Could you check a few things on this model? Use its own coordinates, in mm. Face numbers are marked on the shaded views. A direction names the side the tool comes from. Coordinates: 2 decimals unless noted, no trailing zeros. Loops run counter-clockwise (first coordinate to the right, second up) from the corner with the lowest first, then second, coordinate; pieces in that order, holes last. Notation, with made-up numbers: M -32.75,7.5 L 2.25,7.5 A11 ccw 2.25,19.5 Z; hole C 10.25,1 d8. An arc over 180 degrees is marked long. Write each question's results on one line, items separated by ' | '.
```python
from build123d import *

# Parameters (mm, degrees)
BOSS_EXTRUDE1_DEPTH      = 54
BOSS_EXTRUDE1_DEPTH_BACK = 46
SKETCH1_R                = 15
BOSS_EXTRUDE3_REACH      = 99.568
SKETCH20_R               = 12.5
SKETCH20_R_2             = 10
SKETCH20_3_R             = 10
CUT_EXTRUDE2_DEPTH       = 20
SKETCH22_R               = 12.5
CUT_EXTRUDE3_DEPTH       = 95
CUT_EXTRUDE6_DEPTH       = 24
CUT_EXTRUDE7_REACH       = 125.735
SKETCH23_R               = 2.435


with BuildPart() as part:
    # Sketch1 → Boss-Extrude1 (new, two sides: drawn at the far end of the back side and taken through both)
    with BuildSketch(Plane.XY.offset(-BOSS_EXTRUDE1_DEPTH_BACK)):
        Circle(SKETCH1_R)
    extrude(amount=BOSS_EXTRUDE1_DEPTH + BOSS_EXTRUDE1_DEPTH_BACK)

    # Loft1: read off the stored shape, not the designer's step
    # Loft1: loft between two sections, ruled curve by curve
    loft1_from = [
        Edge.make_line((-13.008298755, 7.468879668, 18.132780083), (-13.008298755, 7.468879668, -18.132780083)),
        Edge.make_line((-13.008298755, 7.468879668, -18.132780083), (13.008298755, 7.468879668, -18.132780083)),
        Edge.make_line((13.008298755, 7.468879668, 18.132780083), (-13.008298755, 7.468879668, 18.132780083)),
        Edge.make_line((13.008298755, 7.468879668, -18.132780083), (13.008298755, 7.468879668, 18.132780083)),
    ]
    loft1_to = [
        Edge.make_line((-7, 30, 12.5), (-7, 30, -12.5)),
        Edge.make_line((-7, 30, -12.5), (7, 30, -12.5)),
        Edge.make_line((7, 30, 12.5), (-7, 30, 12.5)),
        Edge.make_line((7, 30, -12.5), (7, 30, 12.5)),
    ]
    loft1 = Solid(Shell([*[Face.make_surface_from_curves(loft1_from[k], loft1_to[k]) for k in range(4)], Face(Wire(loft1_from)), Face(Wire(loft1_to))]))
    add(loft1)

    # Boss-Extrude3: up to this plane
    boss_extrude3_end = Plane(origin=(-14.004149378, 3.734439834, 0), z_dir=(0.9662349396012463, -0.25766265056033255, 0))
    # Sketch20 → Boss-Extrude3 (add, up to the surface)
    with BuildSketch(Plane(origin=(32.065513698, 51.244565683, 0), x_dir=(0, 0, -1), z_dir=(0.9063077870366495, 0.4226182617407006, 0)), mode=Mode.PRIVATE) as boss_extrude3_sk1:
        with Locations(Location((0, 0, 0), (0, 0, 90))):
            Circle(SKETCH20_R)
        Circle(SKETCH20_R_2, mode=Mode.SUBTRACT)
    boss_extrude3_tool1 = split(extrude(boss_extrude3_sk1.sketch, amount=-BOSS_EXTRUDE3_REACH, mode=Mode.PRIVATE), bisect_by=boss_extrude3_end, keep=Keep.BOTH, mode=Mode.PRIVATE)
    add(boss_extrude3_tool1.solids().sort_by_distance((37.198824, 40.236147, 0))[0])
    # Sketch20 → Boss-Extrude3 (add, up to the surface)
    with BuildSketch(Plane(origin=(32.065513698, 51.244565683, 0), x_dir=(0, 0, -1), z_dir=(0.9063077870366495, 0.4226182617407006, 0)), mode=Mode.PRIVATE) as boss_extrude3_sk2:
        Circle(SKETCH20_R_2)
    boss_extrude3_tool2 = split(extrude(boss_extrude3_sk2.sketch, amount=-BOSS_EXTRUDE3_REACH, mode=Mode.PRIVATE), bisect_by=boss_extrude3_end, keep=Keep.BOTH, mode=Mode.PRIVATE)
    add(boss_extrude3_tool2.solids().sort_by_distance((32.065514, 51.244566, 0))[0])

    # Sketch20<3> → Cut-Extrude2 (cut)
    with BuildSketch(Plane(origin=(32.065513698, 51.244565683, 0), x_dir=(0, 0, -1), z_dir=(0.9063077870366495, 0.4226182617407006, 0))):
        with Locations(Location((0, 0, 0), (0, 0, 90))):
            Circle(SKETCH20_3_R)
    extrude(amount=-CUT_EXTRUDE2_DEPTH, mode=Mode.SUBTRACT)

    # Sketch22 → Cut-Extrude3 (cut)
    with BuildSketch(Plane(origin=(0, 0, -46), x_dir=(-1, 0, 0), z_dir=(0, 0, -1))):
        Circle(SKETCH22_R)
    extrude(amount=-CUT_EXTRUDE3_DEPTH, mode=Mode.SUBTRACT)

    # Sketch22<3> → Cut-Extrude6 (cut)
    with BuildSketch(Plane(origin=(0, 0, -46), x_dir=(-1, 0, 0), z_dir=(0, 0, -1))):
        with BuildLine():
            ThreePointArc((12.5, 0), (0, -12.5), (-12.5, 0))
            Line((-12.5, 0), (-15, 0))
            ThreePointArc((-15, 0), (0, -15), (15, 0))
            Line((15, 0), (12.5, 0))
        make_face()
    extrude(amount=-CUT_EXTRUDE6_DEPTH, mode=Mode.SUBTRACT)

    # Sketch23 → Cut-Extrude7 (cut, up to next)
    with BuildSketch(Plane.XY.offset(54), mode=Mode.PRIVATE) as cut_extrude7_sk1:
        with Locations((2.172182, -4.201728854)):
            Circle(SKETCH23_R)
    cut_extrude7_tool1 = extrude(cut_extrude7_sk1.sketch, amount=-CUT_EXTRUDE7_REACH, mode=Mode.PRIVATE) & part.part
    add(cut_extrude7_tool1.solids().sort_by_distance((2.172182, -4.201729, 54))[0], mode=Mode.SUBTRACT)


with BuildPart() as body_2:
    # Mirror1: mirrored copy
    add(part.part.mirror(Plane.XY.offset(54)))


solid = body_2.part
```
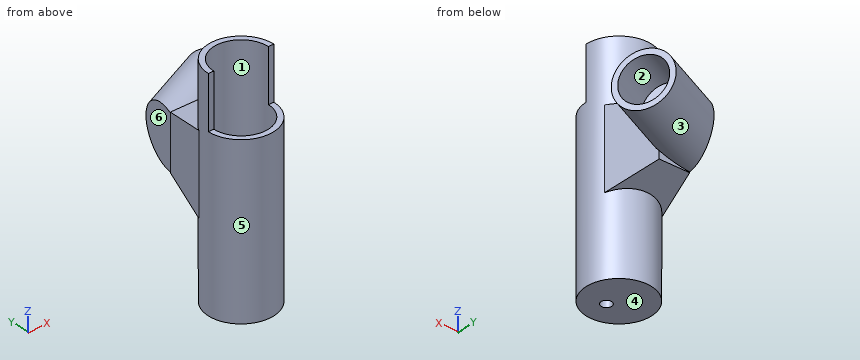
(1) If we mould it in two halves opening along X, with no side actions, what happens to the marked faces 1, 2, 3 and 4? For each: released by +X, released by -X, zero draft, split by the parting line, or undercut.
Reported:
face 1: undercut | face 2: undercut | face 3: split by the parting line | face 4: zero draft
(2) Please list where these lines run through material, in increasing order: probe 1 along Y at (x, z) = (0, 84); probe 2 along X at (y, z) = (-2, 115.5). Write a range as from..to.
Reported:
probe 1: y = -15..-12.5, 12.5..15 | probe 2: x = -14.87..-12.34, 12.34..14.87
(3) Imagine slicing it at A-A, the plane y = 4.5. List the corners of the cut face in (x, z) for me.
Reported:
outline: M -14.31,54 L 14.31,54 L 14.31,154 L 11.66,154 L 11.66,59 L -11.66,59 L -11.66,154 L -14.31,154 Z
(4) Which directions (+Z, -Z, +X, -X, +Y, -Y) give clear straight access to the entire face, cutting with the end or side of a thin tool? Please do the marked faces 5 and 6.
Reported:
face 5: none | face 6: +Z, -Z, -X, +Y
(5) Will these pins go through, and if not, where does the flat tip stop? P1, Ø20, axis at x = 0, y = 0, coming from the +Z side; P2, Ø1, axis at y = 2.5, z = 71, coming from the +X side; P3, Ø1.2, axis at x = 14, z = 148, coming from the -Y side; P4, Ø4, axis at x = 2.17, y = -4.2, coming from the -Z side.
Reported:
P1: stops at z = 59 | P2: stops at x = 14.87 | P3: stops at y = 0 | P4: passes through
(6) Imagine slicing it at B-B, the plane z = 147. List the corners of the cut face in (x, y) for me.
Reported:
outline: M -15,0 L -12.5,0 A12.5 cw 12.5,0 L 15,0 A15 ccw Z
